Geometry check sheet. Reference: the model listing, model coordinates, mm. A direction names the side the tool comes from. Give positions to 0.01 mm unless a question says otherwise; leave off trailing zeros. Write each loop counter-clockwise with the first axis right and the second up, starting at its lowest first coordinate (ties: lowest second). Pieces come first, ordered by that corner, then holes. Notation, with made-up numbers: (12, -17) -> (25, -17) arc R36 cw to (25, 18) -> close; hole circle Ø3 at (57.25, 81.25). An arc over 180 degrees is marked (long way). One line per item, written item: value.
from build123d import *

# Parameters (mm, degrees)
SKETCH1_W           = 3
SKETCH1_H           = 7
SKETCH1_W_2         = 35
SKETCH1_H_2         = 1.2
BOSS_EXTRUDE1_DEPTH = 3


with BuildPart() as part:
    # Sketch1 → Boss-Extrude1 (new body)
    with BuildSketch(Plane(origin=(0, 0, 0), x_dir=(1, 0, 0), z_dir=(0, 1, 0))):
        Polygon((35, 42), (17.5, 42), (17.5, 0), (35, 0), (35, 7), (35, 14), (35, 21), (35, 28), (35, 35), align=None)
        with Locations((36.5, 31.5)):
            Rectangle(SKETCH1_W, SKETCH1_H)
        with Locations((36.5, 17.5)):
            Rectangle(SKETCH1_W, SKETCH1_H)
        with Locations((36.5, 3.5)):
            Rectangle(SKETCH1_W, SKETCH1_H)
        Polygon((17.5, 0), (17.5, 42), (0, 42), (0, 35), (0, 28), (0, 21), (0, 14), (0, 7), (0, 0), align=None)
        with Locations((17.5, -0.6)):
            Rectangle(SKETCH1_W_2, SKETCH1_H_2)
        with Locations((-1.5, 3.5)):
            Rectangle(SKETCH1_W, SKETCH1_H)
        with Locations((-1.5, 17.5)):
            Rectangle(SKETCH1_W, SKETCH1_H)
        with Locations((-1.5, 31.5)):
            Rectangle(SKETCH1_W, SKETCH1_H)
    extrude(amount=BOSS_EXTRUDE1_DEPTH)


solid = part.part
1) Sectioned sample at A-A on y = 1.3. Record the cut outline in (x, z).
Verdict:
outline: (-3, -35) -> (0, -35) -> (0, -42) -> (35, -42) -> (35, -35) -> (38, -35) -> (38, -28) -> (35, -28) -> (35, -21) -> (38, -21) -> (38, -14) -> (35, -14) -> (35, -7) -> (38, -7) -> (38, 0) -> (35, 0) -> (35, 1.2) -> (0, 1.2) -> (0, 0) -> (-3, 0) -> (-3, -7) -> (0, -7) -> (0, -14) -> (-3, -14) -> (-3, -21) -> (0, -21) -> (0, -28) -> (-3, -28) -> close
2) Mould release check, pull along Z, two halves, no side actions. Record for faces 1 (the flat face through (-2, 1, -14)), 2 (the flat face through (18, 1, -42)), 3 (the flat face through (-3, 1, -17)): released by +Z, released by -Z, zero draft, split by the parting line, or undercut.
Verdict:
face 1: undercut
face 2: released by -Z
face 3: zero draft
3) Sectioned sample at B-B on z = -35.5. Record the cut outline in (x, y), plus the area to 3 significant figures.
Verdict:
outline: (0, 0) -> (35, 0) -> (35, 3) -> (0, 3) -> close
area: 105 mm^2
4) Tool access check on faces 4 (the flat face through (0, 1, -25)), 5 (the flat face through (36, 1, -21)), 6 (the flat face through (0, 1, -39)). Record the directions out of +Z, -Z, +X, -X, +Y, -Y that give a thin tool (end or side, any length) a straight path to the whole face; none if there is none.
Verdict:
face 4: -X, +Y, -Y
face 5: +X, +Y, -Y
face 6: -Z, -X, +Y, -Y
5) Scan lines: probe 1 along Z at (x, y) = (-1, 2.65); probe 2 along X at (y, z) = (1.05, -25). Record each from-to range of solid material in increasing order.
Verdict:
probe 1: -35 to -28, -21 to -14, -7 to 0
probe 2: 0 to 35
6) Depth check by flat-ended pin: pin 1 Ø0.9 at (x, y) = (36.5, 1.5) entering from -Z; pin 2 Ø0.6 at (y, z) = (1, 0.5) entering from -X; pin 3 Ø1.5 at (x, y) = (36.5, 1) entering from +Z. Enter the tip coordinate at first touch or a pass-through.
Verdict:
pin 1: z = -35
pin 2: x = 0
pin 3: z = 0
